Part model, mm, in its own coordinate system. A direction names the side the tool comes from. Give positions to 0.01 mm unless a question says otherwise; leave off trailing zeros. Write each loop counter-clockwise with the first axis right and the second up, starting at its lowest first coordinate (ties: lowest second). Pieces come first, ordered by that corner, then holes. Notation, with made-up numbers: M 55.5,69 L 63.5,69 A19 cw 63.5,99 Z; hole C 8,81.5 d2. An arc over 180 degrees is marked long. Answer as CSV lines item,"result". Start each with the question number.
Item 1: Band-saw the part on A-A, the plane z = -96. List the corners of the cut face in (x, y).
Item 2: Band-saw the part on D-D, the plane y = 13. List the corners of the cut face in (x, z), then the cut area to 3 significant figures.
Item 3: Band-saw the part on C-C, the plane z = -32. List the corners of the cut face in (x, y).
Item 4: Band-saw the part on B-B, the plane y = -15. List the corners of the cut face in (x, z).
Item 5: Pin check, flat tips, straight feed: pin 1 (5 mm diameter, centred on y = 30.5, z = -135.5, fed in from -X); pin 2 (1.5 mm diameter, centred on x = -1, y = 6, fed in from -Z); pin 3 (2 mm diameter, centred on x = -2, y = 12, fed in from -Z); pin 4 (1.2 mm diameter, centred on x = -2.5, y = 23.5, fed in from -Z). Stop position of each tip, or through.
Item 6: 3-axis set-ups, long thin cutter, end or side, ignore diameter. For faces 5 (the cylindrical face through (-2.028, 35.859, -113.797)), 6 (the flat face through (0, 14, -123)): which of +Z, -Z, +X, -X, +Y, -Y reach the whole face in a straight line?
Item 7: Two-plate mould, pull along Z, no slides. Class faces 1 (the cylindrical face through (-2.028, 35.859, -45.797)), 2 (the flat face through (-2, 15, -12)), 3 (the flat face through (-2, -25, -123)), 4 (the flat face through (-2.03, 14.44, -250.84)): +Z half, -Z half, draft (parallel to the pull), parting line (faces both ways), or undercut.
Item 8: Wall check: L1, parallel to Y at x = -2.4, z = -218; L2, parallel to Z at x = -1.8, y = -4; L3, parallel to Z at x = -0.8, y = 16. Give the ranges that are in metal, low to high. Write a range as from..to.
from build123d import *

# Parameters (mm, degrees)
SKETCH_1_W          = 4
SKETCH_1_H          = 80
EXTRUDE_3_DEPTH     = 250
EXTRUDE_4_DEPTH     = 80
EXTRUDE_5_DEPTH     = 80
SKETCH_8_W          = 35
SKETCH_8_H          = 44
SKETCH_8_W_2        = 48
CUT_EXTRUDE_1_DEPTH = 258.627972648
SKETCH_2_R          = 2.5
CUT_EXTRUDE_2_DEPTH = 258.627972648
FILLET_1_R          = 4
FILLET_2_R          = 4
FILLET_3_R          = 4
FILLET_4_R          = 4


with BuildPart() as part:
    # 草图1 → 拉伸3 (new body)
    with BuildSketch(Plane.XY):
        with Locations((-2, 15)):
            Rectangle(SKETCH_1_W, SKETCH_1_H)
    extrude(amount=-EXTRUDE_3_DEPTH)

    # 草图4 → 拉伸4 (add)
    with BuildSketch(Plane.XZ.offset(25)):
        Polygon((-4, 0), (-4, 1.656854249), (0, 0), align=None)
    extrude(amount=-EXTRUDE_4_DEPTH)

    # 草图6 → 拉伸5 (add)
    with BuildSketch(Plane.XZ.offset(25)):
        Polygon((-4, -250), (-4, -251.656854249), (0, -250), align=None)
    extrude(amount=-EXTRUDE_5_DEPTH)

    # 草图8 → 切除-拉伸1 (cut, through all)
    with BuildSketch(Plane(origin=(0, 0, 0), x_dir=(0, 0, -1), z_dir=(1, 0, 0))):
        with Locations((29.5, 15)):
            Rectangle(SKETCH_8_W, SKETCH_8_H)
        with Locations((91, 15)):
            Rectangle(SKETCH_8_W_2, SKETCH_8_H)
        with Locations((159, 15)):
            Rectangle(SKETCH_8_W_2, SKETCH_8_H)
        with Locations((220.5, 15)):
            Rectangle(SKETCH_8_W, SKETCH_8_H)
    extrude(amount=-CUT_EXTRUDE_1_DEPTH, mode=Mode.SUBTRACT)

    # 草图2 → 切除-拉伸2 (cut, through all)
    with BuildSketch(Plane.ZY.offset(4)):
        with Locations(Location((-198, 40, 0), (0, 0, 270))):
            Circle(SKETCH_2_R)
        with Locations(Location((-218, -15, 0), (0, 0, 270))):
            Circle(SKETCH_2_R)
        with Locations(Location((-52, 40, 0), (0, 0, 270))):
            Circle(SKETCH_2_R)
        with Locations(Location((-32, -15, 0), (0, 0, 270))):
            Circle(SKETCH_2_R)
    extrude(amount=-CUT_EXTRUDE_2_DEPTH, mode=Mode.SUBTRACT)

    # 圆角1
    fillet_1_edges = [part.edges().sort_by_distance(p)[0] for p in [
        (-2, -7, -12),
        (-2, 37, -12),
        (-2, 37, -47),
        (-2, -7, -47),
    ]]
    fillet(fillet_1_edges, radius=FILLET_1_R)

    # 圆角2
    fillet_2_edges = [part.edges().sort_by_distance(p)[0] for p in [
        (-2, -7, -67),
        (-2, 37, -67),
        (-2, 37, -115),
        (-2, -7, -115),
    ]]
    fillet(fillet_2_edges, radius=FILLET_2_R)

    # 圆角3
    fillet_3_edges = [part.edges().sort_by_distance(p)[0] for p in [
        (-2, -7, -135),
        (-2, 37, -135),
        (-2, 37, -183),
        (-2, -7, -183),
    ]]
    fillet(fillet_3_edges, radius=FILLET_3_R)

    # 圆角4
    fillet_4_edges = [part.edges().sort_by_distance(p)[0] for p in [
        (-2, -7, -203),
        (-2, 37, -203),
        (-2, 37, -238),
        (-2, -7, -238),
    ]]
    fillet(fillet_4_edges, radius=FILLET_4_R)


solid = part.part
Output:
1,outline,"M -4,-25 L 0,-25 L 0,-7 L -4,-7 Z; M -4,37 L 0,37 L 0,55 L -4,55 Z"
2,outline,"M -4,-251.66 L 0,-250 L 0,-238 L -4,-238 Z; M -4,-203 L 0,-203 L 0,-183 L -4,-183 Z; M -4,-135 L 0,-135 L 0,-115 L -4,-115 Z; M -4,-67 L 0,-67 L 0,-47 L -4,-47 Z; M -4,-12 L 0,-12 L 0,0 L -4,1.66 Z"
2,area,"343 mm²"
3,outline,"M -4,-25 L 0,-25 L 0,-17.5 L -4,-17.5 Z; M -4,-12.5 L 0,-12.5 L 0,-7 L -4,-7 Z; M -4,37 L 0,37 L 0,55 L -4,55 Z"
4,outline,"M -4,-251.66 L 0,-250 L 0,-220.5 L -4,-220.5 Z; M -4,-215.5 L 0,-215.5 L 0,-34.5 L -4,-34.5 Z; M -4,-29.5 L 0,-29.5 L 0,0 L -4,1.66 Z"
5,pin 1,"x = -4"
5,pin 2,"z = -250.72"
5,pin 3,"z = -251.24"
5,pin 4,"z = -251.28"
6,face 5,"+X, -X"
6,face 6,"+Z, -Z, +X, +Y, -Y"
7,face 1,"undercut"
7,face 2,"undercut"
7,face 3,"draft"
7,face 4,"-Z half"
8,L1,"-25..-17.5, -12.5..-7, 37..55"
8,L2,"-250.75..-237.87, -203.13..-182.87, -135.13..-114.87, -67.13..-46.87, -12.13..0.75"
8,L3,"-250.33..-238, -203..-183, -135..-115, -67..-47, -12..0.33"
